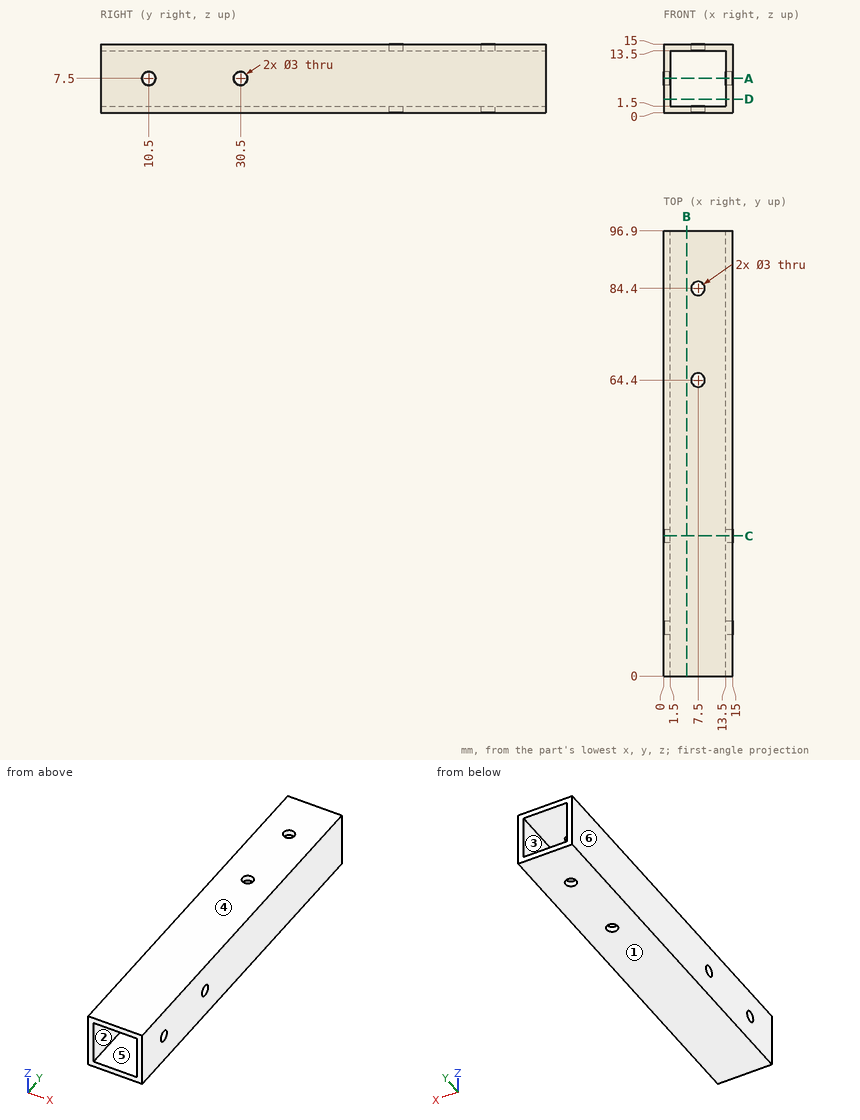
Here's the drawing with two shaded views (mm, measured from the low corner). I have some questions. A direction names the side the tool comes from. Coordinates: 2 decimals unless noted, no trailing zeros. Write each loop counter-clockwise with the first axis right and the second up, starting at its lowest first coordinate (ties: lowest second). Pieces come first, ordered by that corner, then holes.
Item 1: On a 3-axis mill with a long thin cutter (end or side, diameter ignored), from which of +Z, -Z, +X, -X, +Y, -Y can I reach the whole of each face in a straight line? I mean the marked faces 1 and 2. Say none if no direction works.
Item 2: I want a section at D-D on z = 3. Write out the boundary of the cut face in (x, y), and give its area (3 significant figures).
Item 3: If I drill on line 1 (Y direction, x = 1.15, z = 7.5); line 2 (X direction, y = 78, z = 13.25), over which ranges is the centre line in solid material (lowest first)?
Item 4: If we mould it in two halves opening along Z, with no side actions, what happens to the marked faces 3, 4, 5 and 6? For each: +Z half, -Z half, draft (parallel to the pull), parting line (faces both ways), or undercut.
Item 5: I want a section at C-C on y = 30.5. Write out the boundary of the cut face in (x, z).
Item 6: I want a section at B-B on x = 5. Write out the boundary of the cut face in (y, z).
Item 7: Will this pin go through, and if not, where does the flat tip stop? pin 1 (2.5 mm diameter, centred on y = 30.5, z = 7.5, fed in from +X).
Item 8: I want a section at A-A on z = 7.5. Write out the boundary of the cut face in (x, y), and give its area (3 significant figures).
Findings below:
1. face 1: -Z, +X, -X, +Y, -Y
1. face 2: +Y, -Y
2. outline: (0, 0) - (1.5, 0) - (1.5, 96.9) - (0, 96.9) - close; (13.5, 0) - (15, 0) - (15, 96.9) - (13.5, 96.9) - close
2. area: 291 mm2
3. line 1: y = 0 to 9, 12 to 29, 32 to 96.9
3. line 2: x = 0 to 1.5, 13.5 to 15
4. face 3: undercut
4. face 4: +Z half
4. face 5: undercut
4. face 6: draft
5. outline: (0, 0) - (15, 0) - (15, 6) - (13.5, 6) - (13.5, 1.5) - (1.5, 1.5) - (1.5, 6) - (0, 6) - close; (0, 9) - (1.5, 9) - (1.5, 13.5) - (13.5, 13.5) - (13.5, 9) - (15, 9) - (15, 15) - (0, 15) - close
6. outline: (0, 0) - (96.9, 0) - (96.9, 1.5) - (0, 1.5) - close; (0, 13.5) - (96.9, 13.5) - (96.9, 15) - (0, 15) - close
7. pin 1: passes through
8. outline: (0, 0) - (1.5, 0) - (1.5, 9) - (0, 9) - close; (0, 12) - (1.5, 12) - (1.5, 29) - (0, 29) - close; (0, 32) - (1.5, 32) - (1.5, 96.9) - (0, 96.9) - close; (13.5, 0) - (15, 0) - (15, 9) - (13.5, 9) - close; (13.5, 12) - (15, 12) - (15, 29) - (13.5, 29) - close; (13.5, 32) - (15, 32) - (15, 96.9) - (13.5, 96.9) - close
8. area: 273 mm2
